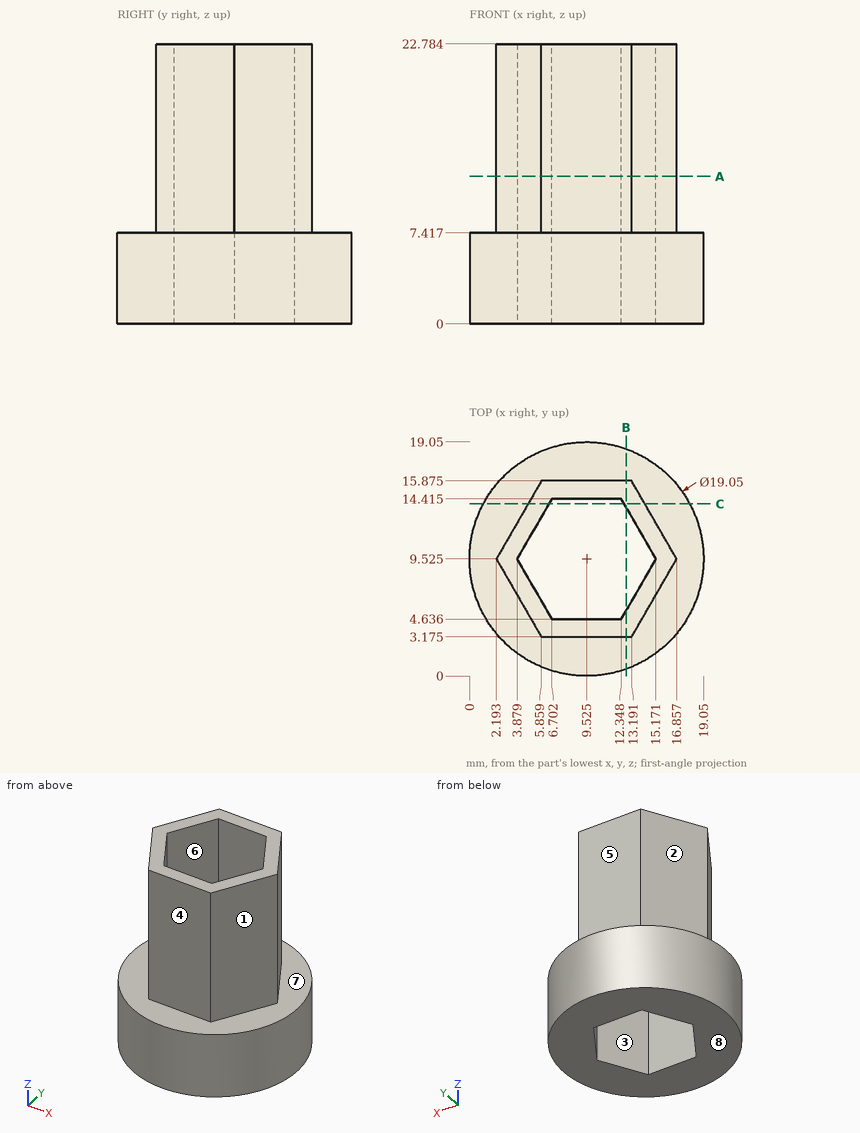
Geometry check sheet. Reference: drawing and pictorial views, mm from the part's lowest x, y, z. A direction names the side the tool comes from. Round coordinates to 2 decimals unless told otherwise and drop trailing zeros. Loops run counter-clockwise (first coordinate to the right, second up) from the corner with the lowest first, then second, coordinate; pieces in that order, holes last. Notation, with made-up numbers: M 52.25,-5.75 L 110.25,-5.75 A27 cw 110.25,30.25 Z; hole C 62.5,-35 d8. An arc over 180 degrees is marked long. One line per item, written item: value.
(1) Thickness scan on line 1 (Y direction, x = 8.25, z = 8.25) (1 decimal); line 2 (Z direction, x = 4.5, y = 13.75); line 3 (X direction, y = 10.25, z = 15.5). Record the ranges inside material, lowest first.
Computed values:
line 1: y = 3.2 to 4.6, 14.4 to 15.9
line 2: z = 0 to 7.42
line 3: x = 2.61 to 4.3, 14.75 to 16.44
(2) Sectioned sample at B-B, the plane x = 12.75. Record the cut outline in (y, z) (1 decimal).
Computed values:
outline: M 0.6,0 L 5.3,0 L 5.3,22.8 L 3.2,22.8 L 3.2,7.4 L 0.6,7.4 Z; M 13.7,0 L 18.5,0 L 18.5,7.4 L 15.9,7.4 L 15.9,22.8 L 13.7,22.8 Z
(3) Depth check by flat-ended pin: pin 1 Ø3 at (x, z) = (10, 10) entering from +Y (1 decimal); pin 2 Ø10 at (x, z) = (3.5, 6.5) entering from +Y (1 decimal); pin 3 Ø10 at (x, y) = (3.5, 12) entering from +Z; pin 4 Ø1 at (x, z) = (3, 12) entering from -Y. Enter the tip coordinate at first touch or a pass-through.
Computed values:
pin 1: stops at y = 15.9
pin 2: stops at y = 19
pin 3: stops at z = 22.78
pin 4: stops at y = 7.26
(4) Access from +Z, -Z, +X, -X, +Y, -Y to the whole of each face (thin tool, end or side, straight path). Record for the marked faces 4, 5, 6, 7 and 8.
Computed values:
face 4: +Z, +X, -X, -Y
face 5: +Z, +X, -X, +Y
face 6: +Z, -Z
face 7: +Z
face 8: -Z, +X, -X, +Y, -Y
(5) Release check for a two-part mould opening along Y. For the marked faces 1, 2 and 3 record: +Y half, -Y half, draft (parallel to the pull), parting line (faces both ways), or undercut.
Computed values:
face 1: -Y half
face 2: +Y half
face 3: undercut
(6) Sectioned sample at A-A, the plane z = 12. Record the cut outline in (x, y) (1 decimal).
Computed values:
outline: M 2.2,9.5 L 5.9,3.2 L 13.2,3.2 L 16.9,9.5 L 13.2,15.9 L 5.9,15.9 Z; hole M 3.9,9.5 L 6.7,4.6 L 12.3,4.6 L 15.2,9.5 L 12.3,14.4 L 6.7,14.4 Z
(7) Sectioned sample at C-C, the plane y = 14. Record the cut outline in (x, z).
Computed values:
outline: M 1.12,0 L 6.46,0 L 6.46,22.78 L 4.78,22.78 L 4.78,7.42 L 1.12,7.42 Z; M 12.59,0 L 17.93,0 L 17.93,7.42 L 14.27,7.42 L 14.27,22.78 L 12.59,22.78 Z
